The drawing under review shows one solid part. Ordinate dimensions are in mm from its lowest x, y, z. A direction names the side the tool comes from. Give positions to 0.01 mm unless a question says otherwise; leave off trailing zeros. Write each loop counter-clockwise with the first axis right and the second up, starting at its lowest first coordinate (ties: lowest second). Pieces come first, ordered by that corner, then holes.
Q1. We need section D-D (z = 13.5). Write out the cut boundary in (x, y), then the cut area to 3 significant figures.
Q2. Machinability: for the marked faces 1, 2 and 3, which of the approach directions +Z, -Z, +X, -X, +Y, -Y give a long, thin tool a straight path to every point of the face, cutting with its end or side? Answer none if there is none.
Q3. We need section A-A (x = 3.2). Write out the cut boundary in (y, z), then the cut area to 3 significant figures.
Q4. We need section B-B (z = 3.2). Write out the cut boundary in (x, y), then the cut area to 3 significant figures.
Q5. Insertion check: P1, Ø8, axis at y = 7, z = 26, coming from the -X side; P2, Ø4.5, axis at x = 66.8, z = 27.9, coming from the -Y side; P3, Ø2, axis at x = 66.8, z = 3.2, coming from the +Y side; P4, Ø4, axis at x = 5, y = 4, coming from the +Z side. Each pin has a flat end and moves straight along its axis. Give the tip position at first contact, or say it passes through.
Q6. For line 1 (X direction, y = 16.3, z = 27.9); line 2 (Z direction, x = 66.8, y = 14.95); line 3 (X direction, y = 4.25, z = 9), list the stretches that pass through material, from the lowest coordinate up.
Q7. We need section C-C (y = 15.5). Write out the cut boundary in (x, z).
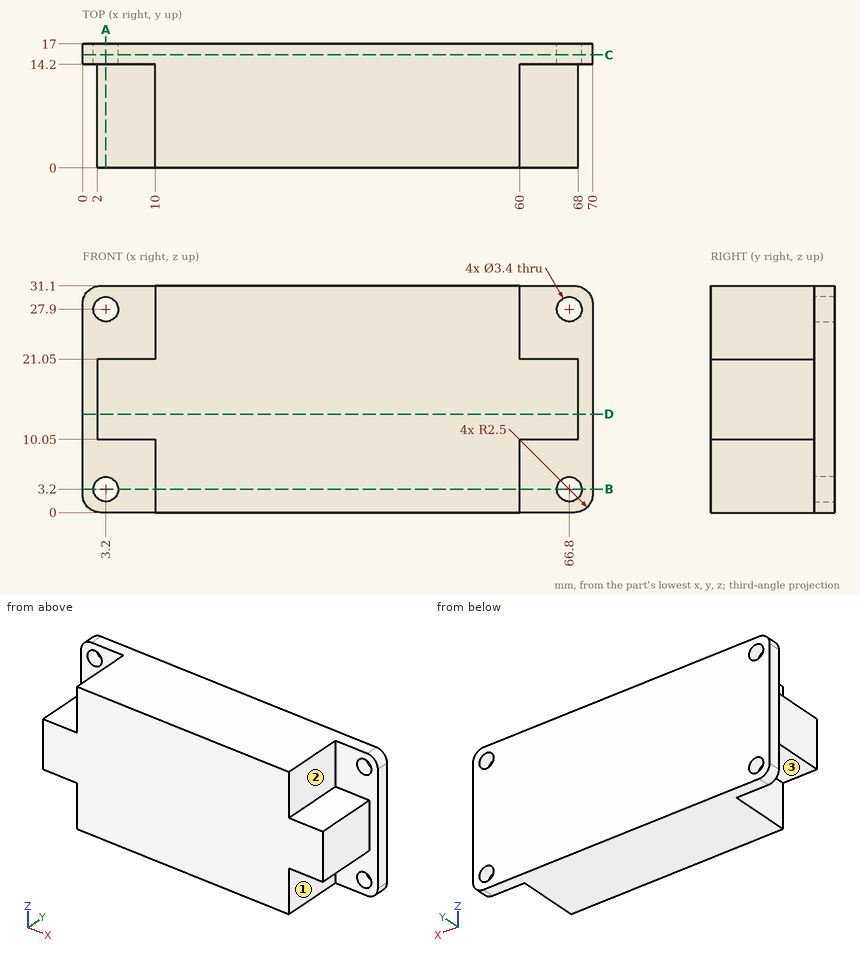
Computed:
1. outline: (0, 14.2) - (2, 14.2) - (2, 0) - (68, 0) - (68, 14.2) - (70, 14.2) - (70, 17) - (0, 17) - close
1. area: 1,130 mm2
2. face 1: -Z, +X, -Y
2. face 2: +Z, +X, -Y
2. face 3: -Z, -X, -Y
3. outline: (0, 10.05) - (14.2, 10.05) - (14.2, 4.9) - (17, 4.9) - (17, 26.2) - (14.2, 26.2) - (14.2, 21.05) - (0, 21.05) - close; (14.2, 0) - (17, 0) - (17, 1.5) - (14.2, 1.5) - close; (14.2, 29.6) - (17, 29.6) - (17, 31.1) - (14.2, 31.1) - close
3. area: 224 mm2
4. outline: (0, 14.2) - (1.5, 14.2) - (1.5, 17) - (0, 17) - close; (4.9, 14.2) - (10, 14.2) - (10, 0) - (60, 0) - (60, 14.2) - (65.1, 14.2) - (65.1, 17) - (4.9, 17) - close; (68.5, 14.2) - (70, 14.2) - (70, 17) - (68.5, 17) - close
4. area: 887 mm2
5. P1: stops at x = 10
5. P2: stops at y = 14.2
5. P3: passes through
5. P4: stops at z = 21.05
6. line 1: x = 0 to 1.5, 4.9 to 65.1, 68.5 to 70
6. line 2: z = 0 to 1.5, 4.9 to 26.2, 29.6 to 31.1
6. line 3: x = 10 to 60
7. outline: (0, 2.5) arc R2.5 ccw to (2.5, 0) - (67.5, 0) arc R2.5 ccw to (70, 2.5) - (70, 28.6) arc R2.5 ccw to (67.5, 31.1) - (2.5, 31.1) arc R2.5 ccw to (0, 28.6) - close; hole circle Ø3.4 at (3.2, 3.2); hole circle Ø3.4 at (3.2, 27.9); hole circle Ø3.4 at (66.8, 3.2); hole circle Ø3.4 at (66.8, 27.9)
